The model under review builds one solid part; all positions refer to its coordinate system, in mm. A direction names the side the tool comes from. Round coordinates to 2 decimals unless told otherwise and drop trailing zeros. Loops run counter-clockwise (first coordinate to the right, second up) from the corner with the lowest first, then second, coordinate; pieces in that order, holes last. Notation, with made-up numbers: M -11.75,25 L 31.25,25 A14 ccw 31.25,48 Z; hole C 66,41.25 d1. An arc over 180 degrees is marked long. Answer in a Markdown table with one row per item. Add a question column.
from build123d import *

# Parameters (mm, degrees)
F1_DEPTH = 20


with BuildPart() as f1:
    # F0 (on Front) → F1 (new body)
    with BuildSketch(Plane.XZ):
        with BuildLine():
            ThreePointArc((489.067735, 244.89684), (-0.249757, 148.374207), (-489.567249, 244.89684))
            ThreePointArc((-489.567249, 244.89684), (-870.956673, 25.346072), (-562.960597, -288.976771))
            ThreePointArc((-562.960597, -288.976771), (-0.249757, -256.22251), (562.461083, -288.976771))
            ThreePointArc((562.461083, -288.976771), (870.457159, 25.346072), (489.067735, 244.89684))
        make_face()
        with BuildLine():
            ThreePointArc((-568.76174, -239.314444), (-821.422552, 18.536454), (-508.554405, 198.642241))
            ThreePointArc((-508.554405, 198.642241), (-0.249757, 98.374207), (508.054891, 198.642241))
            ThreePointArc((508.054891, 198.642241), (820.923038, 18.536454), (568.262226, -239.314444))
            ThreePointArc((568.262226, -239.314444), (-0.249757, -206.22251), (-568.76174, -239.314444))
        make_face(mode=Mode.SUBTRACT)
    extrude(amount=F1_DEPTH)


solid = f1.part
1. Mouldability with a two-part tool opening along X and no side actions: class faces 1 (the cylindrical face through (-822.143, -9.86, 12.752)), 2 (the flat face through (60, -20, 112)) as released by +X, released by -X, zero draft, split by the parting line, or undercut.
2. Machinability: for faces 3 (the cylindrical face through (6.777, -9.86, 148.393)), 4 (the cylindrical face through (7.73, -9.86, -206.23)), which of the approach directions +Z, -Z, +X, -X, +Y, -Y give a long, thin tool a straight path to every point of the face, cutting with its end or side? Answer none if there is none.
3. For pin 1 Ø3 at (y, z) = (-17, 190.5) entering from -X; pin 2 Ø2 at (y, z) = (-2.5, 198.5) entering from +X, all flat-tipped, find the tip position at first contact; note any pin that passes through.
4. Take a section at C-C, the plane y = -9.5. State the section outline as (x, z) points.
5. Take a section at A-A, the plane x = -725.5. State the section outline as (y, z) points, and give its area (3 significant figures).
6. To check wall thickness, follow probe 1 along Z at (x, y) = (-696, -6.5); probe 2 along X at (y, z) = (-2, -193.5); probe 3 along Z at (x, y) = (392, -17). State the ranges of each line that lie inside material, in increasing order.
7. Take a section at B-B, the plane z = -184. State the section outline as (x, y) points, and give its area (3 significant figures).
Check sheet entries:
| question | item | result |
|---|---|---|
| 1 | face 1 | undercut |
| 1 | face 2 | zero draft |
| 2 | face 3 | +Z, +Y, -Y |
| 2 | face 4 | +Y, -Y |
| 3 | pin 1 | stops at x = -787.15 |
| 3 | pin 2 | stops at x = 777.31 |
| 4 | outline | M -562.96,-288.98 A4850 cw 562.46,-288.98 A278.3 ccw long 489.07,244.9 A1288.55 cw -489.57,244.9 A278.3 ccw long Z; hole M -568.76,-239.31 A4900 cw 568.26,-239.31 A228.3 ccw long 508.05,198.64 A1338.55 cw -508.55,198.64 A228.3 ccw long Z |
| 5 | outline | M -20,-258.49 L 0,-258.49 L 0,-200.05 L -20,-200.05 Z; M -20,174.94 L 0,174.94 L 0,233.38 L -20,233.38 Z |
| 5 | area | 2,340 mm^2 |
| 6 | probe 1 | z = -271.98 to -217.42, 192.31 to 246.87 |
| 6 | probe 2 | x = -806.7 to -734.46, 733.96 to 806.2 |
| 6 | probe 3 | z = -272.11 to -221.95, 157.14 to 209.53 |
| 7 | outline | M -814.47,-20 L -746.01,-20 L -746.01,0 L -814.47,0 Z; M 745.51,-20 L 813.97,-20 L 813.97,0 L 745.51,0 Z |
| 7 | area | 2,740 mm^2 |
